Geometry: final body of the model. Coordinates: model frame, mm. Round coordinates to 2 decimals unless told otherwise and drop trailing zeros. Write each loop counter-clockwise with the first axis right and the second up, starting at its lowest first coordinate (ties: lowest second). Pieces come first, ordered by that corner, then holes. Notation, with made-up numbers: M 68,-23 L 118,-23 A25 cw 118,3 Z; hole C 52,73 d6. An arc over 180 degrees is marked long. Use one line per item in the form item = value. Start each with the question number.
Item 1: Section query A-A (z = 0.6). Return loops of the section in (x, y).
Item 2: Section query C-C (y = 18). Return loops of the section in (x, z), and give its area (3 significant figures).
Item 3: Section query B-B (x = -2). Return loops of the section in (y, z), and give its area (3 significant figures).
Item 4: Pin query (flat end, axial travel): pin 1 Ø1.5 at (y, z) = (39.5, 2.5) entering from -X; pin 2 Ø3 at (x, y) = (-16, 38) entering from -Z. Return the tip coordinate at first contact, or that it passes through.
Item 5: Ray query, probe 1 along Y at (x, z) = (-30, 2.05); probe 2 along X at (y, z) = (31, 1.1); probe 3 along X at (y, z) = (20.5, 2.95). Return the intervals inside material, ascending.
from build123d import *

# Parameters (mm, degrees)
F1_DEPTH = 3.048


with BuildPart() as f1:
    # F0 (on Top) → F1 (new body)
    with BuildSketch(Plane.XY):
        with BuildLine():
            Line((-27.485451, 10.792716), (-29.787896, 42.739153))
            ThreePointArc((-29.787896, 42.739153), (-41.382102, 37.543924), (-45.561652, 25.546117))
            ThreePointArc((-45.561652, 25.546117), (-39.704821, 14.271652), (-27.485451, 10.792716))
        make_face()
        Polygon((0, 32.953762), (-29.787896, 42.739153), (-27.485451, 10.792716), (0, 19.139083), align=None)
        with BuildLine():
            ThreePointArc((0, 19.139083), (9.557615, 26.046422), (0, 32.953762))
            Line((0, 32.953762), (0, 19.139083))
        make_face()
    extrude(amount=F1_DEPTH)


solid = f1.part
Working result:
q1.outline = M -45.56,25.55 A16.04 ccw -27.49,10.79 L 0,19.14 A7.27 ccw long 0,32.95 L -29.79,42.74 A16.04 ccw Z
q2.outline = M -43.04,0 L -3.75,0 L -3.75,3.05 L -43.04,3.05 Z
q2.area = 120 mm²
q3.outline = M 18.53,0 L 33.61,0 L 33.61,3.05 L 18.53,3.05 Z
q3.area = 46.0 mm²
q4.pin_1 = -40.15
q4.pin_2 = 0
q5.probe_1 = 10.66 to 42.73
q5.probe_2 = -45.02 to 7.61
q5.probe_3 = -44.36 to 6.99
